Geometry: final body of the model. Coordinates: model frame, mm. Face numbers are marked on the shaded views. A direction names the side the tool comes from. Give positions to 0.01 mm unless a question says otherwise; leave off trailing zeros. Write each loop counter-clockwise with the first axis right and the second up, starting at its lowest first coordinate (ties: lowest second). Pieces come first, ordered by that corner, then holes. Notation, with made-up numbers: (43, -34) - (88, -34) arc R17 ccw to (88, -19) - close; hole circle Ø9 at (-11, -2.75). An arc over 180 degrees is marked (long way). Return JSON: item names as keys, results as strings.
from build123d import *

# Parameters (mm, degrees)
SKETCH1_R           = 32
MOTORBODY_DEPTH     = 99.6
SKETCH2_R           = 15
MOTORAXLE_DEPTH     = 66
SKETCH3_W           = 65
SKETCH3_H           = 58.4
GEARBOX_DEPTH       = 64
SKETCH4_R           = 5
BOSS_EXTRUDE4_DEPTH = 50.6
SKETCH5_R           = 12.375
SKETCH5_R_2         = 10.375
BOSS_EXTRUDE5_DEPTH = 3.6
SKETCH6_R           = 2
CUT_EXTRUDE1_DEPTH  = 10
BOSS_EXTRUDE6_DEPTH = 15
CUT_EXTRUDE2_DEPTH  = 1.5
SKETCH10_R          = 1.95
SKETCH10_R_2        = 1.5
CUT_EXTRUDE3_DEPTH  = 9.5
SKETCH11_W          = 65
SKETCH11_H          = 64
SKETCH11_R          = 25.7
CUT_EXTRUDE4_DEPTH  = 5.5
SKETCH12_R          = 2.5
CUT_EXTRUDE5_DEPTH  = 13
SKETCH13_R          = 2.5
CUT_EXTRUDE11_DEPTH = 12.75
SKETCH14_R          = 2.5
CUT_EXTRUDE12_DEPTH = 10


with BuildPart() as part:
    # Sketch1 → MotorBody (new body)
    with BuildSketch(Plane(origin=(0, 0, 0), x_dir=(0, 0, -1), z_dir=(1, 0, 0))):
        Circle(SKETCH1_R)
    extrude(amount=MOTORBODY_DEPTH)

    # Sketch2 → MotorAxle (add)
    with BuildSketch(Plane.ZY):
        Circle(SKETCH2_R)
    extrude(amount=MOTORAXLE_DEPTH)

    # Sketch3 → Gearbox (add)
    with BuildSketch(Plane.XY):
        with Locations((-33.5, 0.8)):
            Rectangle(SKETCH3_W, SKETCH3_H)
    extrude(amount=GEARBOX_DEPTH)

    # Sketch4 → Boss-Extrude4 (add)
    with BuildSketch(Plane.XZ.offset(28.4)):
        with Locations((-31, 29)):
            Circle(SKETCH4_R)
    extrude(amount=BOSS_EXTRUDE4_DEPTH)

    # Sketch5 → Boss-Extrude5 (add)
    with BuildSketch(Plane.XZ.offset(28.4)):
        with Locations((-31, 29)):
            Circle(SKETCH5_R)
        with Locations((-31, 29)):
            Circle(SKETCH5_R_2, mode=Mode.SUBTRACT)
    extrude(amount=BOSS_EXTRUDE5_DEPTH)

    # Sketch6 → Cut-Extrude1 (cut)
    with BuildSketch(Plane.XZ.offset(79)):
        with Locations((-31, 29)):
            Circle(SKETCH6_R)
    extrude(amount=-CUT_EXTRUDE1_DEPTH, mode=Mode.SUBTRACT)

    # Sketch7 → Boss-Extrude6 (add)
    with BuildSketch(Plane(origin=(99.6, 0, 0), x_dir=(0, 0, -1), z_dir=(1, 0, 0))):
        with BuildLine():
            Line((-31.318365081, 6.56962774), (6.56962774, -31.318365081))
            ThreePointArc((6.56962774, -31.318365081), (22.627416998, -22.627416998), (31.318365081, -6.56962774))
            Line((31.318365081, -6.56962774), (-6.56962774, 31.318365081))
            ThreePointArc((-6.56962774, 31.318365081), (-22.627416998, 22.627416998), (-31.318365081, 6.56962774))
        make_face()
    extrude(amount=BOSS_EXTRUDE6_DEPTH)

    # Sketch9 → Cut-Extrude2 (cut, symmetric)
    with BuildSketch(Plane.XY.offset(29)):
        with BuildLine():
            Line((-26, -64), (-26, -52))
            ThreePointArc((-26, -52), (-29.6, -58), (-26, -64))
        make_face()
    extrude(amount=CUT_EXTRUDE2_DEPTH, both=True, mode=Mode.SUBTRACT)

    # Sketch10 → Cut-Extrude3 (cut)
    with BuildSketch(Plane.XZ.offset(28.4)):
        with Locations((-45.142135624, 43.142135624)):
            Circle(SKETCH10_R)
        with Locations((-16.857864376, 43.142135624)):
            Circle(SKETCH10_R)
        with Locations((-16.857864376, 14.857864376)):
            Circle(SKETCH10_R)
        with Locations((-45.142135624, 14.857864376)):
            Circle(SKETCH10_R)
        with Locations((-31, 49)):
            Circle(SKETCH10_R_2)
        with Locations((-11, 29)):
            Circle(SKETCH10_R_2)
        with Locations((-51, 29)):
            Circle(SKETCH10_R_2)
        with Locations((-31, 9)):
            Circle(SKETCH10_R_2)
    extrude(amount=-CUT_EXTRUDE3_DEPTH, mode=Mode.SUBTRACT)

    # Sketch11 → Cut-Extrude4 (cut)
    with BuildSketch(Plane.XZ.offset(28.4)):
        with Locations((-33.5, 32)):
            Rectangle(SKETCH11_W, SKETCH11_H)
        with Locations((-31, 29)):
            Circle(SKETCH11_R, mode=Mode.SUBTRACT)
    extrude(amount=-CUT_EXTRUDE4_DEPTH, mode=Mode.SUBTRACT)

    # Sketch12 → Cut-Extrude5 (cut)
    with BuildSketch(Plane.XZ.offset(22.9)):
        with Locations((-56, 49)):
            Circle(SKETCH12_R)
        with Locations((-6, 49)):
            Circle(SKETCH12_R)
        with Locations((-6, 9)):
            Circle(SKETCH12_R)
        with Locations((-56, 9)):
            Circle(SKETCH12_R)
    extrude(amount=-CUT_EXTRUDE5_DEPTH, mode=Mode.SUBTRACT)

    # Sketch13 → Cut-Extrude11 (cut)
    with BuildSketch(Plane.XY.offset(64)):
        with Locations((-56, 14.3)):
            Circle(SKETCH13_R)
        with Locations((-6, 14.3)):
            Circle(SKETCH13_R)
        with Locations((-56, -15.7)):
            Circle(SKETCH13_R)
        with Locations((-6, -15.7)):
            Circle(SKETCH13_R)
    extrude(amount=-CUT_EXTRUDE11_DEPTH, mode=Mode.SUBTRACT)

    # Sketch14 → Cut-Extrude12 (cut)
    with BuildSketch(Plane.ZY.offset(66)):
        with Locations((4.091432188, 14.3)):
            Circle(SKETCH14_R)
        with Locations((54.091432188, 14.3)):
            Circle(SKETCH14_R)
        with Locations((4.091432188, -15.7)):
            Circle(SKETCH14_R)
        with Locations((54.091432188, -15.7)):
            Circle(SKETCH14_R)
    extrude(amount=-CUT_EXTRUDE12_DEPTH, mode=Mode.SUBTRACT)


solid = part.part
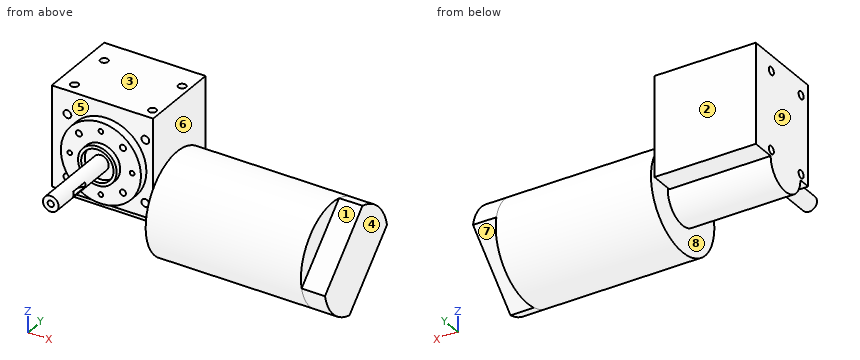
Q1. Material intervals for probe 1 along Y at (x, z) = (-56, 60); probe 2 along Z at (x, y) = (-11, -22); probe 3 along X at (y, z) = (21.5, 10), sorted ascending. Write a range as [from, to].
Answer key:
{"probe 1": "y = [-22.9, -18.2], [-13.2, 11.8], [16.8, 30]", "probe 2": "z = [0, 27.5], [30.5, 64]", "probe 3": "x = [-66, -1], [0, 114.6]"}
Q2. Section query C-C, the plane x = -24. Return the cut outline in (y, z).
Answer key:
{"outline": "(-32, 18.8) - (-28.4, 18.8) - (-28.4, 4.27) - (-22.9, 4.27) - (-22.9, 0) - (-15, 0) arc R15 ccw to (15, 0) - (30, 0) - (30, 64) - (-22.9, 64) - (-22.9, 53.73) - (-28.4, 53.73) - (-28.4, 39.2) - (-32, 39.2) - (-32, 36.66) - (-28.4, 36.66) - (-28.4, 21.34) - (-32, 21.34) - close"}
Q3. Section query B-B, the plane x = 61. Return the cut outline in (y, z), plus the area to 3 significant figures.
Answer key:
{"outline": "circle Ø64 at (0, 0)", "area": "3,220 mm^2"}
Q4. Section query D-D, the plane y = -48. Return the cut outline in (x, z).
Answer key:
{"outline": "circle Ø10 at (-31, 29)"}
Q5. Set-up query: the marked faces 1, 2, 3, 4 and 5. Return all of +Z, -Z, +X, -X, +Y, -Y with unobstructed straight access to the full face (end or side cutting, diameter ignored); none if empty.
Answer key:
{"face 1": "+Z, +X, -Y", "face 2": "+Z, -Z, -X, +Y", "face 3": "+Z, +X, -X, +Y, -Y", "face 4": "+Z, -Z, +X, +Y, -Y", "face 5": "-Y"}
Q6. Pin query (flat end, axial travel): P1, Ø2, axis at x = 24.5, z = 1.5, coming from the -Y side; P2, Ø6, axis at x = 46.5, y = -28.5, coming from the +Z side; P3, Ø12, axis at x = -24, z = 26.5, coming from the +Y side. Return the tip coordinate at first contact, or that it passes through.
Answer key:
{"P1": "stops at y = -32", "P2": "stops at z = 19.33", "P3": "stops at y = 30"}
Q7. Mould query, pull axis X, two halves, no side actions, for the marked faces 6, 7, 8 and 9. Classes: pulls with the +X half, pulls with the -X half, needs draft (parallel to the pull), parting line crosses it, or undercut.
Answer key:
{"face 6": "undercut", "face 7": "needs draft", "face 8": "undercut", "face 9": "pulls with the -X half"}
Q8. Section query A-A, the plane y = 0. Return the cut outline in (x, z).
Answer key:
{"outline": "(-66, -15) - (0, -15) - (0, -32) - (99.6, -32) - (99.6, -24.75) - (114.6, -24.75) - (114.6, 24.75) - (99.6, 24.75) - (99.6, 32) - (0, 32) - (0, 15) - (-1, 15) - (-1, 64) - (-66, 64) - close"}
